Here's how the part is built. I have some questions about the finished solid (model axes, mm). A direction names the side the tool comes from. Coordinates: 2 decimals unless noted, no trailing zeros. Loops run counter-clockwise (first coordinate to the right, second up) from the corner with the lowest first, then second, coordinate; pieces in that order, holes last. Notation, with made-up numbers: (33.5, -15.5) -> (75.5, -15.5) arc R28 cw to (75.5, 4.5) -> close; hole circle Ø6 at (82, -32). An arc over 180 degrees is marked (long way). Answer as a JSON object with one key per item and string values. Group by question number.
1) I want a section at B-B (z = 4). Write out the boundary of the cut face in (x, y).
2) I want a section at A-A (y = -15.5). Write out the boundary of the cut face in (x, z), then the cut area to 3 significant figures.
3) I need wall thicknesses on probe 1 along X at (y, z) = (-30.5, 5); probe 2 along X at (y, z) = (-36.5, 9.25); probe 3 along Z at (x, y) = (-9, -42.5). Which ranges of each line are inside material? Lowest first, please. Write a range as [from, to].
4) I'm going to push flat-ended pins straight in: pin 1 (3 mm diameter, centred on y = -41.5, z = 6.5, fed in from -X); pin 2 (1.3 mm diameter, centred on x = -15.5, z = 6.5, fed in from -Y); pin 3 (1 mm diameter, centred on y = 18.5, z = 10.5, fed in from -X). Where does each tip first touch, or does it pass through?
5) Which directions (+Z, -Z, +X, -X, +Y, -Y) give clear straight access to the entire face, cutting with the end or side of a thin tool? Please do faces 4 (the flat face through (10.363, -30, 6)), 5 (the flat face through (-13.12, 2.58, 10.2)), 6 (the cylindrical face through (8.915, -26.2, 1.528)), 7 (the flat face through (13.05, 2.58, 10.2)).
6) If we mould it in two halves opening along X, with no side actions, what happens to faces 1 (the flat face through (-8.1, 27, 10.2)), 2 (the flat face through (7.788, -27.089, 10.196)), 3 (the flat face through (0, -6, 0))? For each: +X half, -X half, draft (parallel to the pull), parting line (faces both ways), or undercut.
```python
from build123d import *

# Parameters (mm, degrees)
F0_W     = 20.116801
F0_H     = 58.369201
F1_DEPTH = 12.7
F2_SIZE  = 5.08
F3_R     = 5.08


with BuildPart() as f1:
    # F0 (on Top) → F1 (new body)
    with BuildSketch(Plane.XY):
        Polygon((21.031201, 0), (0, 55.016398), (-21.336, 0), (-9.753601, 0), (10.3632, 0), align=None)
        with Locations((0.304799, -29.1846)):
            Rectangle(F0_W, F0_H)
    extrude(amount=F1_DEPTH)

    # F2
    f2_edges = [f1.edges().sort_by_distance(p)[0] for p in [
        (10.5156, 27.508199, 12.7),
        (-10.668, 27.508199, 12.7),
        (-15.544801, 0, 12.7),
        (-9.753601, -29.1846, 12.7),
        (0.3048, -58.369201, 12.7),
        (10.3632, -29.1846, 12.7),
        (15.6972, 0, 12.7),
    ]]
    chamfer(f2_edges, length=F2_SIZE)

    # F3
    f3_edges = [f1.edges().sort_by_distance(p)[0] for p in [
        (10.5156, 27.508199, 0),
        (-10.668, 27.508199, 0),
        (-15.544801, 0, 0),
        (-9.753601, -29.1846, 0),
        (0.3048, -58.369201, 0),
        (10.3632, -29.1846, 0),
        (15.6972, 0, 0),
    ]]
    fillet(f3_edges, radius=F3_R)


solid = f1.part
```
Determined:
{
 "1": {"outline": "(-21.17, 0.12) -> (-9.64, 0.12) -> (-9.64, -58.25) -> (10.25, -58.25) -> (10.25, 0.12) -> (20.86, 0.12) -> (0, 54.69) -> close"},
 "2": {"outline": "(-9.75, 5.08) arc R5.08 ccw to (-4.67, 0) -> (5.28, 0) arc R5.08 ccw to (10.36, 5.08) -> (10.36, 7.62) -> (5.28, 12.7) -> (-4.67, 12.7) -> (-9.75, 7.62) -> close", "area": "219 mm^2"},
 "3": {"probe 1": "[-9.75, 10.36]", "probe 2": "[-8.12, 8.73]", "probe 3": "[2.42, 8.37]"},
 "4": {"pin 1": "x = -9.75", "pin 2": "y = 0", "pin 3": "x = -11.64"},
 "5": {"face 4": "+Z, -Z, +X, -Y", "face 5": "+Z, -X, -Y", "face 6": "-Z, +X, -Y", "face 7": "+Z, +X, -Y"},
 "6": {"face 1": "-X half", "face 2": "+X half", "face 3": "draft"}
}
